Model file for the job. Use its own axes, mm. Face numbers are marked on the shaded views. A direction names the side the tool comes from. Round coordinates to 2 decimals unless told otherwise and drop trailing zeros. Write each loop counter-clockwise with the first axis right and the second up, starting at its lowest first coordinate (ties: lowest second). Pieces come first, ordered by that corner, then holes. Notation, with made-up numbers: (30, 27.5) - (43, 27.5) arc R9 ccw to (43, 42.5) - close; hole circle Ø6 at (-6, 31). An arc over 180 degrees is marked (long way). Answer as a JSON object with one key per item and string values. Group by question number.
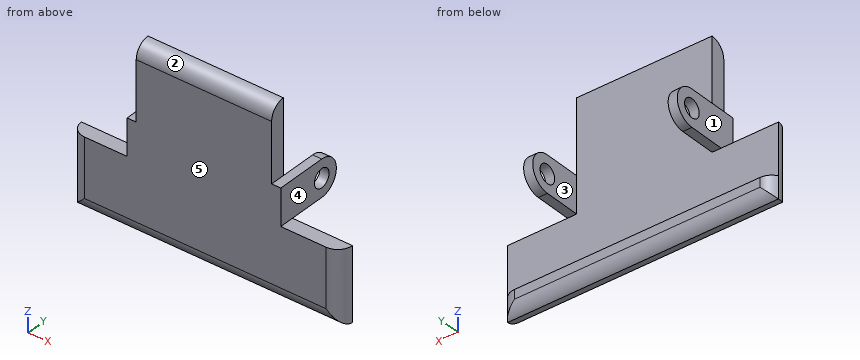
from build123d import *

# Parameters (mm, degrees)
F1_DEPTH     = 5.08
F2_R         = 5.07999
F3_R         = 3.175
F3_W         = 5.08
F3_H         = 12.7
F4_DEPTH     = 3.175
F5_R         = 3.175
F5_W         = 5.08
F5_H         = 12.7
F6_DEPTH     = 3.175
F7_W         = 94.3114114086
F7_H         = 7.62
F8_DEPTH     = 2.54
F9_T1_DEPTH  = 116.3084855321
F9_T6_DEPTH  = 29.6170741236
F9_T11_DEPTH = 29.6170741236


# Not quite as in the source:
# - a fillet or chamfer that OpenCascade refuses, or shapes differently, is made with other operations: its cross-section is extruded or revolved along the edge and cut away or added
# - a fillet or chamfer is up to 0.001 mm smaller than in the source, because OpenCascade refuses the exact size


with BuildPart() as f1:
    # F0 (on Front) → F1 (new body)
    with BuildSketch(Plane.XZ):
        Polygon((-23.1219715205, 38.3847513186), (-23.1219715205, 0), (-46.243943041, 0), (-46.243943041, -25.4), (48.0674683675, -25.4), (48.0674683675, 0), (24.0337341838, 0), (24.0337341838, 38.3847513186), align=None)
    extrude(amount=F1_DEPTH)

    # F2 (radius 5.08 in the source; OpenCascade refuses exactly that, so slightly less here)
    f2_edges = [f1.edges().sort_by_distance(p)[0] for p in [
        (-46.243943, -5.08, -12.7),
        (48.067468, -5.08, -12.7),
        (0.911763, -5.08, -25.4),
        (0.455881, -5.08, 38.384751),
    ]]
    fillet(f2_edges, radius=F2_R)

    # F3 (on face) → F4 (join)
    with BuildSketch(Plane(origin=(-23.1219715205, 0, 0), x_dir=(0, -1, 0), z_dir=(-1, 0, 0))):
        with BuildLine():
            Line((-12.7, 0), (0, 0))
            Line((0, 0), (0, 12.7))
            Line((0, 12.7), (-12.7, 12.7))
            ThreePointArc((-12.7, 12.7), (-19.05, 6.35), (-12.7, 0))
        make_face()
        with Locations((-12.7, 6.35)):
            Circle(F3_R, mode=Mode.SUBTRACT)
        with Locations((2.54, 6.35)):
            Rectangle(F3_W, F3_H)
    extrude(amount=F4_DEPTH)

    # F5 (on face) → F6 (join)
    with BuildSketch(Plane.YZ.offset(24.0337341838)):
        with BuildLine():
            Line((0, 12.7), (0, 0))
            Line((0, 0), (12.7, 0))
            ThreePointArc((12.7, 0), (19.05, 6.35), (12.7, 12.7))
            Line((12.7, 12.7), (0, 12.7))
        make_face()
        with Locations((12.7, 6.3747640323)):
            Circle(F5_R, mode=Mode.SUBTRACT)
        with Locations((-2.54, 6.35)):
            Rectangle(F5_W, F5_H)
    extrude(amount=F6_DEPTH)

    # F7 (on face) → F8 (join)
    with BuildSketch(Plane(origin=(0, 0, 0), x_dir=(-1, 0, 0), z_dir=(0, 1, 0))):
        with Locations((-0.9117626632, -21.59)):
            Rectangle(F7_W, F7_H)
    extrude(amount=F8_DEPTH)

    # F9: fillet of radius 5.08 on 3 edges, made by hand

    # F9_s2 → F9_t1 (cut)
    with BuildSketch(Plane.YZ.offset(-57.2424801028)):
        with BuildLine():
            ThreePointArc((-1e-05, -25.4), (1.8594061645, -23.5405901753), (2.54, -21.0005851753))
            Line((2.54, -21.0005851753), (2.54, -25.4))
            Line((2.54, -25.4), (-1e-05, -25.4))
        make_face()
    extrude(amount=F9_T1_DEPTH, mode=Mode.SUBTRACT)


with BuildPart() as f9_tool4:
    # F9_s5 → F9_t6 (new body)
    with BuildSketch(Plane.XY.offset(-36.3985370618)):
        with BuildLine():
            ThreePointArc((-46.243943041, -1e-05), (-44.3845332163, 1.8594061645), (-41.8445282163, 2.54))
            Line((-41.8445282163, 2.54), (-46.243943041, 2.54))
            Line((-46.243943041, 2.54), (-46.243943041, -1e-05))
        make_face()
    extrude(amount=F9_T6_DEPTH)

    split(bisect_by=Plane.XZ, keep=Keep.BOTTOM)


with BuildPart() as f1_1:
    add(f1.part)

    # F9_t3: cut F9_tool4
    add(f9_tool4.part, mode=Mode.SUBTRACT)


with BuildPart() as f9_tool9:
    # F9_s10 → F9_t11 (new body)
    with BuildSketch(Plane.XY.offset(-6.7814629382)):
        with BuildLine():
            ThreePointArc((43.6680535428, 2.54), (46.2080585428, 1.8594061645), (48.0674683675, -1e-05))
            Line((48.0674683675, -1e-05), (48.0674683675, 2.54))
            Line((48.0674683675, 2.54), (43.6680535428, 2.54))
        make_face()
    extrude(amount=-F9_T11_DEPTH)

    split(bisect_by=Plane.XZ, keep=Keep.BOTTOM)


with BuildPart() as f1_2:
    add(f1_1.part)

    # F9_t8: cut F9_tool9
    add(f9_tool9.part, mode=Mode.SUBTRACT)


solid = f1_2.part
(1) Slice it at B-B (y = 11.75). Write the cut outline in (x, z).
(2) Pull direction X, two halves, no side cores. Call the marked faces 1, 2 and 3: pulls with the +X half, pulls with the -X half, needs draft (parallel to the pull), parting line crosses it, or undercut.
(3) Drill centre lines: line 1 (Z direction, x = 25.5, y = 12.7); line 2 (X direction, y = 16.75, z = 10); line 3 (Y direction, x = -25, z = 6). Where is each one in solid material? Low to high. Write a range as from..to.
(4) 3-axis set-ups, long thin cutter, end or side, ignore diameter. For the marked faces 4 and 5: which of +Z, -Z, +X, -X, +Y, -Y reach the whole face in a straight line?
(5) Slice it at A-A (x = 34). Write the cut outline in (y, z), then the cut area to 3 significant figures.
(6) Flat gauge pins, fed straight in: pin 1 (5.5 mm diameter, centred on y = -2.5, z = 20.5, fed in from +X); pin 2 (6.5 mm diameter, centred on y = 11.5, z = 5, fed in from +X); pin 3 (2.5 mm diameter, centred on x = 25.5, y = 6, fed in from +Z). Where does each tip first touch, or does it go through?
(7) Slice it at D-D (y = -1.75). Write the cut outline in (x, z), then the cut area to 3 significant figures.
Answer:
{
 "1": {"outline": "(-26.3, 0) - (-23.12, 0) - (-23.12, 3.32) - (-26.3, 3.32) - close; (-26.3, 9.38) - (-23.12, 9.38) - (-23.12, 12.7) - (-26.3, 12.7) - close; (24.03, 0) - (27.21, 0) - (27.21, 3.35) - (24.03, 3.35) - close; (24.03, 9.4) - (27.21, 9.4) - (27.21, 12.7) - (24.03, 12.7) - close"},
 "2": {"face 1": "pulls with the -X half", "face 2": "needs draft", "face 3": "undercut"},
 "3": {"line 1": "0..3.2, 9.55..12.7", "line 2": "-26.3..-23.12, 24.03..27.21", "line 3": "-5.08..9.54, 15.86..19.04"},
 "4": {"face 4": "+Z, +X, +Y, -Y", "face 5": "+Z, -Z, +X, -X, -Y"},
 "5": {"outline": "(-5.08, -20.32) arc R5.08 ccw to (0, -25.4) arc R5.08 ccw to (2.54, -21) - (2.54, -17.78) - (0, -17.78) - (0, 0) - (-5.08, 0) - close", "area": "140 mm²"},
 "6": {"pin 1": "x = 24.03", "pin 2": "x = 27.21", "pin 3": "z = 12.7"},
 "7": {"outline": "(-45.93, -25.09) - (47.76, -25.09) - (47.76, 0) - (27.21, 0) - (27.21, 12.7) - (24.03, 12.7) - (24.03, 38.07) - (-23.12, 38.07) - (-23.12, 12.7) - (-26.3, 12.7) - (-26.3, 0) - (-45.93, 0) - close", "area": "4,230 mm²"}
}
